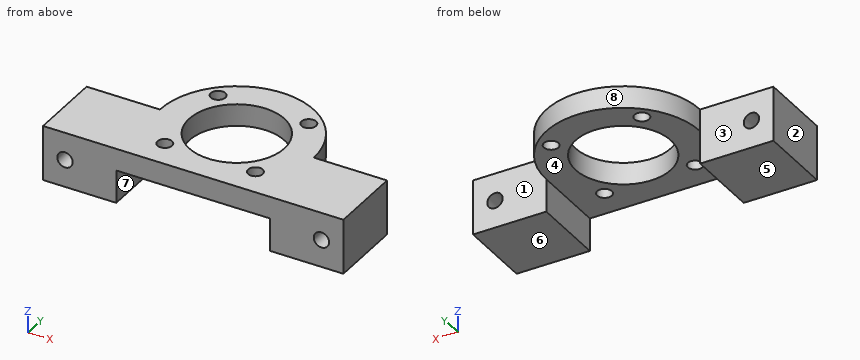
from build123d import *

# Parameters (mm, degrees)
SKETCH_1_R          = 13
SKETCH_1_R_2        = 2
EXTRUDE_1_DEPTH     = 6
SKETCH_2_W          = 20
SKETCH_2_H          = 20.22
EXTRUDE_2_DEPTH     = 15
SKETCH_3_R          = 2.1
CUT_EXTRUDE_1_DEPTH = 47.936126811


with BuildPart() as part:
    # 草图1 → 凸台-拉伸1 (new body)
    with BuildSketch(Plane.XY):
        with BuildLine():
            Line((-21, 20.22), (-21, 0))
            Line((-21, 0), (21, 0))
            Line((21, 0), (21, 20.22))
            ThreePointArc((21, 20.22), (0, 41.22), (-21, 20.22))
        make_face()
        with Locations((0, 20.22)):
            Circle(SKETCH_1_R, mode=Mode.SUBTRACT)
        with Locations((-12.374368671, 32.594368671)):
            Circle(SKETCH_1_R_2, mode=Mode.SUBTRACT)
        with Locations((12.374368671, 32.594368671)):
            Circle(SKETCH_1_R_2, mode=Mode.SUBTRACT)
        with Locations((12.374368671, 7.845631329)):
            Circle(SKETCH_1_R_2, mode=Mode.SUBTRACT)
        with Locations((-12.374368671, 7.845631329)):
            Circle(SKETCH_1_R_2, mode=Mode.SUBTRACT)
    extrude(amount=EXTRUDE_1_DEPTH)

    # 草图2 → 凸台-拉伸2 (add)
    with BuildSketch(Plane.XY.offset(6)):
        with Locations((-31, 10.11)):
            Rectangle(SKETCH_2_W, SKETCH_2_H)
        with Locations((31, 10.11)):
            Rectangle(SKETCH_2_W, SKETCH_2_H)
    extrude(amount=-EXTRUDE_2_DEPTH)

    # 草图3 → 切除-拉伸1 (cut, through all)
    with BuildSketch(Plane(origin=(0, 20.22, 0), x_dir=(1, 0, 0), z_dir=(0, 1, 0))):
        with Locations(Location((-35, 1.5, 0), (0, 0, 180))):
            Circle(SKETCH_3_R)
        with Locations((35, 1.5)):
            Circle(SKETCH_3_R)
    extrude(amount=-CUT_EXTRUDE_1_DEPTH, mode=Mode.SUBTRACT)


solid = part.part
Can you work these out from the model? Positions are in its coordinate system, mm. Face numbers are marked on the shaded views. A direction names the side the tool comes from. Coordinates: 2 decimals unless noted, no trailing zeros. Loops run counter-clockwise (first coordinate to the right, second up) from the corner with the lowest first, then second, coordinate; pieces in that order, holes last. Notation, with made-up numbers: (2.5, 88.25) - (20.5, 88.25) arc R21 cw to (20.5, 116.25) - close; hole circle Ø2 at (5, 59). An arc over 180 degrees is marked (long way). Put each result on its own line as item: value. Start each with the question number.
Item 1: If I drill on line 1 along Z through (x, y) = (35, 17.5); line 2 along Y through (x, z) = (0, 3.05); line 3 along Y through (x, z) = (12, 1.75), over which ranges is the centre line in solid material (lowest first)?
Item 2: Suppose I cut it at A-A (x = -35). Please give me the cut outline in (y, z).
Item 3: Suppose I cut it at C-C (y = 9). Please give me the cut outline in (x, z).
Item 4: Suppose I cut it at B-B (z = -7.5). Please give me the cut outline in (x, y).
Item 5: Which directions (+Z, -Z, +X, -X, +Y, -Y) give clear straight access to the entire face, cutting with the end or side of a thin tool? Please do the marked faces 1, 2, 3, 4 and 5.
Item 6: Suppose I cut it at D-D (y = 14). Please give me the cut outline in (x, z), and give its area (3 significant figures).
Item 7: If we mould it in two halves opening along X, with no side actions, what happens to the marked faces 6, 7 and 8? For each: +X half, -X half, draft (parallel to the pull), parting line (faces both ways), or undercut.
Item 8: For pin 1 (6.5 mm diameter, centred on x = 12.37, y = 7.85, fed in from -Z); pin 2 (4.5 mm diameter, centred on x = 28, z = 1.5, fed in from +Y), each with a flat end and sliding along its axis, tell me the tip position at first contact or that it passes through.
Here are the results:
1. line 1: -9 to -3.6, 0.6 to 6
1. line 2: 0 to 7.22, 33.22 to 41.22
1. line 3: 0 to 5.88, 9.81 to 15.22, 25.22 to 30.63, 34.56 to 37.45
2. outline: (0, -9) - (20.22, -9) - (20.22, -3.6) - (0, -3.6) - close; (0, 0.6) - (20.22, 0.6) - (20.22, 6) - (0, 6) - close
3. outline: (-41, -9) - (-21, -9) - (-21, 0) - (-14.01, 0) - (-14.01, 6) - (-41, 6) - close; (-10.74, 0) - (-6.57, 0) - (-6.57, 6) - (-10.74, 6) - close; (6.57, 0) - (10.74, 0) - (10.74, 6) - (6.57, 6) - close; (14.01, 0) - (21, 0) - (21, -9) - (41, -9) - (41, 6) - (14.01, 6) - close; hole circle Ø4.2 at (-35, -1.5); hole circle Ø4.2 at (35, -1.5)
4. outline: (-41, 0) - (-21, 0) - (-21, 20.22) - (-41, 20.22) - close; (21, 0) - (41, 0) - (41, 20.22) - (21, 20.22) - close
5. face 1: +Z, -Z, +X, +Y
5. face 2: +Z, -Z, -X, +Y, -Y
5. face 3: +Z, -Z, -X, +Y
5. face 4: -Z, +Y, -Y
5. face 5: -Z, +X, -X, +Y, -Y
6. outline: (-41, -9) - (-21, -9) - (-21, 0) - (-11.42, 0) - (-11.42, 6) - (-41, 6) - close; (11.42, 0) - (21, 0) - (21, -9) - (41, -9) - (41, 6) - (11.42, 6) - close; hole circle Ø4.2 at (-35, -1.5); hole circle Ø4.2 at (35, -1.5)
6. area: 687 mm²
7. face 6: draft
7. face 7: undercut
7. face 8: parting line
8. pin 1: z = 0
8. pin 2: y = 20.22
